Here's how the part is built. I have some questions about the finished solid (model axes, mm). Face numbers are marked on the shaded views. A direction names the side the tool comes from. Coordinates: 2 decimals unless noted, no trailing zeros. Order: outer loops, then holes, each group sorted by start corner. A loop starts at its lowest first (then second) coordinate and runs counter-clockwise, first axis right, second up. Notation, with made-up numbers: (41, 19.25) - (92, 19.25) arc R21 ccw to (92, 49.25) - close; hole circle Ø3 at (59.25, 13.5). An arc over 180 degrees is marked (long way). Use one line per item in the form item = value. Start each with the question number.
from build123d import *

# Parameters (mm, degrees)
F0_W     = 12
F0_H     = 12
F1_DEPTH = 3.5
F2_R     = 4
F3_DEPTH = 1.5
F4_R     = 0.75
F5_DEPTH = 1.5
F6_W     = 1.3371782843
F6_H     = 0.1306298655


with BuildPart() as f1:
    # F0 (on Top) → F1 (new body)
    with BuildSketch(Plane.XY):
        Rectangle(F0_W, F0_H)
    extrude(amount=-F1_DEPTH)

    # F2 (on Top) → F3 (cut)
    with BuildSketch(Plane.XY):
        Circle(F2_R)
    extrude(amount=-F3_DEPTH, mode=Mode.SUBTRACT)

    # F4 (on face) → F5 (join)
    with BuildSketch(Plane(origin=(0, 0, -3.5), x_dir=(1, 0, 0), z_dir=(0, 0, -1))):
        with Locations((0, -3.75)):
            Circle(F4_R)
        with Locations((0, 3.75)):
            Circle(F4_R)
    extrude(amount=F5_DEPTH)

    # F8: sweep along a path in F7
    with BuildLine(Plane(origin=(0, 6, 0), x_dir=(-1, 0, 0), z_dir=(0, 1, 0))) as f8_path:
        ThreePointArc((-6, -2.9808722661), (-6.2386599526, -3.0614322815), (-6.3796732575, -3.2701515593))
        Line((-6.3796732575, -3.2701515593), (-6.7573431879, -4.6420912258))
        ThreePointArc((-6.7573431879, -4.6420912258), (-6.7854382425, -4.8500061966), (-6.7573431879, -5.0579211675))
        Line((-6.7573431879, -5.0579211675), (-6.3840173786, -6.4140801969))
    # F6 (on face) → F8 (sweep)
    with BuildSketch(Plane.YZ.offset(6)):
        with Locations((-3.7832342787, -3.070783685)):
            Rectangle(F6_W, F6_H)
        with Locations((3.7832342787, -3.070783685)):
            Rectangle(F6_W, F6_H)
    sweep(path=f8_path.line)

    # F9: F1 across plane


with BuildPart() as f1_1:
    add(f1.part)
    add(f1.part.mirror(Plane.YZ))


solid = f1_1.part
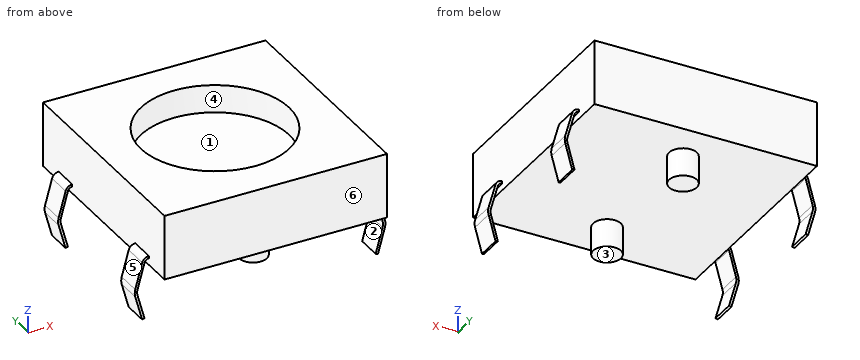
1) I need wall thicknesses on probe 1 along Y at (x, z) = (0, -0.4); probe 2 along Z at (x, y) = (-2.75, 5.25). Which ranges of each line are inside material? Lowest first, please. Write a range as [from, to].
2) Suppose I cut it at A-A, the plane y = 0. List the corners of the cut face in (x, z) for me.
3) For pin 1 (7 mm diameter, centred on x = 0, y = 0, fed in from -Z); pin 2 (0.6 mm diameter, centred on x = 6.5, z = -4, fed in from -Y); pin 3 (0.8 mm diameter, centred on x = 6.5, z = -5.5, fed in from +Y), each with a flat end and sliding along its axis, tell me the tip position at first contact or that it passes through.
4) Suppose I cut it at B-B, the plane x = 0. List the corners of the cut face in (y, z) for me.
5) If we mould it in two halves opening along X, with no side actions, what happens to the marked faces 4, 5 and 6? For each: pulls with the +X half, pulls with the -X half, needs draft (parallel to the pull), parting line crosses it, or undercut.
6) Which directions (+Z, -Z, +X, -X, +Y, -Y) give clear straight access to the entire face, cutting with the end or side of a thin tool? Please do the marked faces 1, 2 and 3.
7) Suppose I cut it at C-C, the plane x = 3.5. List the corners of the cut face in (y, z) for me.
From the geometry:
q1.probe_1 = [-6, -4], [4, 6]
q1.probe_2 = [-3.5, 0]
q2.outline = (-6, -3.5) - (6, -3.5) - (6, 0) - (4, 0) - (4, -1.5) - (-4, -1.5) - (-4, 0) - (-6, 0) - close
q3.pin_1 = -5
q3.pin_2 = -4.45
q3.pin_3 = 4.45
q4.outline = (-6, -3.5) - (-4.5, -3.5) - (-4.5, -5) - (-3, -5) - (-3, -3.5) - (3, -3.5) - (3, -5) - (4.5, -5) - (4.5, -3.5) - (6, -3.5) - (6, 0) - (4, 0) - (4, -1.5) - (-4, -1.5) - (-4, 0) - (-6, 0) - close
q5.face_4 = undercut
q5.face_5 = pulls with the -X half
q5.face_6 = needs draft
q6.face_1 = +Z
q6.face_2 = +Y, -Y
q6.face_3 = -Z, +Y, -Y
q7.outline = (-6, -3.5) - (6, -3.5) - (6, 0) - (1.94, 0) - (1.94, -1.5) - (-1.94, -1.5) - (-1.94, 0) - (-6, 0) - close
